Work out the finished part from the listing and answer in its coordinate system (mm). A direction names the side the tool comes from. Round coordinates to 2 decimals unless told otherwise and drop trailing zeros. Write each loop counter-clockwise with the first axis right and the second up, starting at its lowest first coordinate (ties: lowest second). Pieces come first, ordered by that corner, then holes. Notation, with made-up numbers: (14, -23.75) -> (67, -23.75) arc R31 cw to (67, 0.25) -> close; hole circle Ø7 at (-6, 79.25). An arc over 180 degrees is marked (long way). Answer as a JSON object with one key per item and string values. Group by question number.
from build123d import *

# Parameters (mm, degrees)
F1_DEPTH = 760
F2_W     = 50
F2_H     = 25
F2_W_2   = 560
F3_DEPTH = 260.001


with BuildPart() as f1:
    # F0 (on Front) → F1 (new body)
    with BuildSketch(Plane.XZ):
        Polygon((115, 70), (-115, 70), (-115, 0), (-100, 0), (-70, 0), (70, 0), (100, 0), (115, 0), align=None)
        Polygon((-70, 0), (-100, 0), (-100, -23.5), (-130, -23.5), (-130, -25), (-95, -25), (-95, -5), (-70, -5), align=None)
        Polygon((100, -23.5), (100, 0), (70, 0), (70, -5), (95, -5), (95, -25), (130, -25), (130, -23.5), align=None)
    extrude(amount=F1_DEPTH)

    # F2 (on face) → F3 (cut, through all)
    with BuildSketch(Plane(origin=(-130, 0, 0), x_dir=(0, -1, 0), z_dir=(-1, 0, 0))):
        with Locations((25, -12.5)):
            Rectangle(F2_W, F2_H)
        with Locations((735, -12.5)):
            Rectangle(F2_W, F2_H)
        with Locations((380, -12.5)):
            Rectangle(F2_W_2, F2_H)
    extrude(amount=-F3_DEPTH, mode=Mode.SUBTRACT)


solid = f1.part
1) For a pull along X with two mould halves and no side action, classify faces 1 (the face through (100, -685, -12)), 2 (the face through (82, -75, -5)), 3 (the face through (115, -685, -23.5)) as released by +X, released by -X, zero draft, split by the parting line, or undercut.
2) Straight lines are drawn through the part: L1, parallel to Z at x = -6, y = -383.5; L2, parallel to X at y = -55, z = -10; L3, parallel to X at y = -34.5, z = 17. For each, find the intervals that lie inside material, in ascending order.
3) Each of these flat-tipped pins is pushed along its axis until it touches: P1, Ø7.5, axis at x = 95.5, z = -9, coming from the -Y side; P2, Ø8, axis at y = -381.5, z = 31.5, coming from the -X side; P3, Ø10, axis at y = -684, z = -19.5, coming from the +X side; P4, Ø7.5, axis at x = -83.5, y = -676, coming from the -Z side. Where does it stop, or does it pass through?
4) A tool of negligible diameter and unlimited length cuts with its end or side. For faces 4 (the face through (-115, -685, -23.5)), 5 (the face through (-95, -685, -15)), 6 (the face through (95.4, -710, -11.6)), 7 (the face through (95.4, -100, -11.6)), from which of +Z, -Z, +X, -X, +Y, -Y can it reach the whole face along a straight path? Write none if from no direction.
5) A cutting plane is placed at C-C on x = -20. Determine the outline of the cut face in (y, z).
6) A cutting plane is placed at A-A on z = -13. Determine the outline of the cut face in (x, y).
7) A cutting plane is placed at D-D on y = -241. Determine the outline of the cut face in (x, z), plus the area to 3 significant figures.
8) A cutting plane is placed at B-B on y = -83.5. Determine the outline of the cut face in (x, z).
Established:
{
 "1": {"face 1": "released by +X", "face 2": "undercut", "face 3": "zero draft"},
 "2": {"L1": "z = 0 to 70", "L2": "x = -100 to -95, 95 to 100", "L3": "x = -115 to 115"},
 "3": {"P1": "stops at y = -710", "P2": "stops at x = -115", "P3": "stops at x = 130", "P4": "stops at z = -5"},
 "4": {"face 4": "-X, +Y, -Y", "face 5": "-Z, +Y, -Y", "face 6": "-Z, +X, -X, -Y", "face 7": "-Z, +X, -X"},
 "5": {"outline": "(-760, 0) -> (0, 0) -> (0, 70) -> (-760, 70) -> close"},
 "6": {"outline": "(-100, -710) -> (-95, -710) -> (-95, -660) -> (-100, -660) -> close; (-100, -100) -> (-95, -100) -> (-95, -50) -> (-100, -50) -> close; (95, -710) -> (100, -710) -> (100, -660) -> (95, -660) -> close; (95, -100) -> (100, -100) -> (100, -50) -> (95, -50) -> close"},
 "7": {"outline": "(-115, 0) -> (115, 0) -> (115, 70) -> (-115, 70) -> close", "area": "16,100 mm²"},
 "8": {"outline": "(-130, -25) -> (-95, -25) -> (-95, -5) -> (-70, -5) -> (-70, 0) -> (70, 0) -> (70, -5) -> (95, -5) -> (95, -25) -> (130, -25) -> (130, -23.5) -> (100, -23.5) -> (100, 0) -> (115, 0) -> (115, 70) -> (-115, 70) -> (-115, 0) -> (-100, 0) -> (-100, -23.5) -> (-130, -23.5) -> close"}
}
